from build123d import *

# Parameters (mm, degrees)
F1_DEPTH = 8
F2_SIZE  = 30
F3_R     = 8
F4_R     = 3
F6_D     = 6.5
F8_D     = 10.5


with BuildPart() as f1:
    # F0 (on Front) → F1 (new body)
    with BuildSketch(Plane.XZ):
        Polygon((-41, 0), (0, 0), (0, 281), (-50, 281), (-50, 278), (-80, 278), (-80, 20), (-41, 20), align=None)
    extrude(amount=F1_DEPTH)

    # F2
    f2_edges = [f1.edges().sort_by_distance(p)[0] for p in [
        (0, -4, 281),
    ]]
    chamfer(f2_edges, length=F2_SIZE)

    # F3
    f3_edges = [f1.edges().sort_by_distance(p)[0] for p in [
        (-30, -4, 281),
        (0, -4, 251),
    ]]
    fillet(f3_edges, radius=F3_R)

    # F4
    f4_edges = [f1.edges().sort_by_distance(p)[0] for p in [
        (-41, -4, 20),
    ]]
    fillet(f4_edges, radius=F4_R)

    # F6 (through all)
    with Locations(Plane.XZ.offset(8)):
        with Locations((-68.65, 197), (-53.65, 197), (-53.65, 147), (-68.65, 147), (-53.65, 97), (-68.65, 97)):
            Hole(F6_D / 2)

    # F8 (through all)
    with Locations(Plane.XZ.offset(8)):
        with Locations((-32.1, 213.1), (-32.1, 8.1)):
            Hole(F8_D / 2)


solid = f1.part
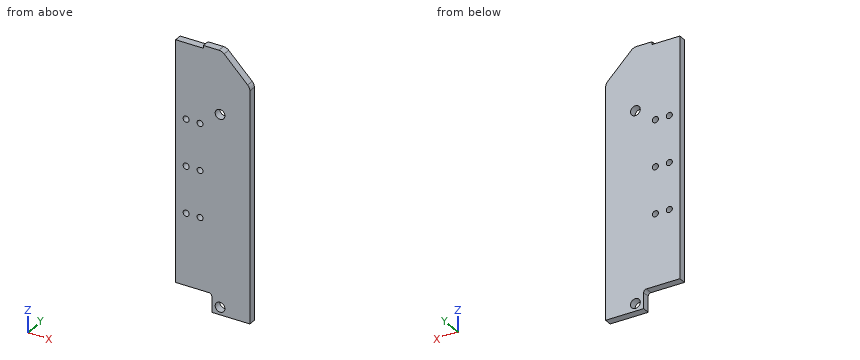
The listing builds one solid part. Answer for the finished solid, in the listing's coordinates (mm). Give positions to 0.01 mm unless a question says otherwise; leave off trailing zeros. Loops run counter-clockwise (first coordinate to the right, second up) from the corner with the lowest first, then second, coordinate; pieces in that order, holes last. Notation, with made-up numbers: (-32.75, -11) - (0.25, -11) arc R8 ccw to (0.25, -6) - close; hole circle Ø11 at (33, -4.75). An arc over 180 degrees is marked (long way). Use one line per item in the form item = value.
1. Section C-C on y = -1.25 is taken. Count the separate pieces of the cut face and the enclosed holes in it, then the cut area to 3 significant figures.
Calculated:
separate_pieces = 1
enclosed_holes = 8
area = 20,800 mm^2
2. Section A-A on z = 97 is taken. Give the vertices of the cut face in (x, y), then the cut area to 3 significant figures.
Calculated:
outline = (-80, -8) - (-71.9, -8) - (-71.9, 0) - (-80, 0) - close; (-65.4, -8) - (-56.9, -8) - (-56.9, 0) - (-65.4, 0) - close; (-50.4, -8) - (0, -8) - (0, 0) - (-50.4, 0) - close
area = 536 mm^2
3. Section D-D on z = 213.1 is taken. Give the vertices of the cut face in (x, y).
Calculated:
outline = (-80, -8) - (-37.35, -8) - (-37.35, 0) - (-80, 0) - close; (-26.85, -8) - (0, -8) - (0, 0) - (-26.85, 0) - close
4. Section B-B on x = -68.65 is taken. Give the vertices of the cut face in (y, z).
Calculated:
outline = (-8, 20) - (0, 20) - (0, 93.75) - (-8, 93.75) - close; (-8, 100.25) - (0, 100.25) - (0, 143.75) - (-8, 143.75) - close; (-8, 150.25) - (0, 150.25) - (0, 193.75) - (-8, 193.75) - close; (-8, 200.25) - (0, 200.25) - (0, 278) - (-8, 278) - close
5. Given pin 1 Ø6 at (x, z) = (-68.65, 97) entering from -Y; pin 2 Ø17 at (x, z) = (-32.1, 8.1) entering from -Y; pin 3 Ø4 at (x, y) = (-12, -5) entering from +Z, each flat-ended and moving along its own axis, determine where each tip first touches the part or whether it passes through.
Calculated:
pin_1 = through
pin_2 = -8
pin_3 = 265
6. Find the intervals of material crossed by line 1 along X through (y, z) = (-2.5, 197); line 2 along Z through (x, y) = (-53.65, -2); line 3 along X through (y, z) = (-2.75, 99), in increasing order. Write a range as [from, to].
Calculated:
line_1 = [-80, -71.9], [-65.4, -56.9], [-50.4, 0]
line_2 = [20, 93.75], [100.25, 143.75], [150.25, 193.75], [200.25, 278]
line_3 = [-80, -71.21], [-66.09, -56.21], [-51.09, 0]
